Geometry check sheet. Reference: drawing and pictorial views, mm from the part's lowest x, y, z. Round coordinates to 2 decimals unless told otherwise and drop trailing zeros. Order: outer loops, then holes, each group sorted by start corner. A loop starts at its lowest first (then second) coordinate and runs counter-clockwise, first axis right, second up.
(1) Cross-section at A-A on y = 10.5. Enter the section's corners in (x, z), and give its area (3 significant figures).
(2) Cross-section at B-B on x = 11.5. Enter the section's corners in (y, z), and give its area (3 significant figures).
(3) Thickness scan on L1, parallel to X at y = 22, z = 55; L2, parallel to Y at x = 54, z = 206.5. Record the ranges inside material, lowest first.
(4) Draft check along Y on the marked faces 1, 2, 3 and 4. Enter one of: pulls with the +Y half, pulls with the -Y half, needs draft (parallel to the pull), parting line crosses it, or undercut.
(5) Cross-section at C-C on z = 185.5. Enter the section's corners in (x, y), and give its area (3 significant figures).
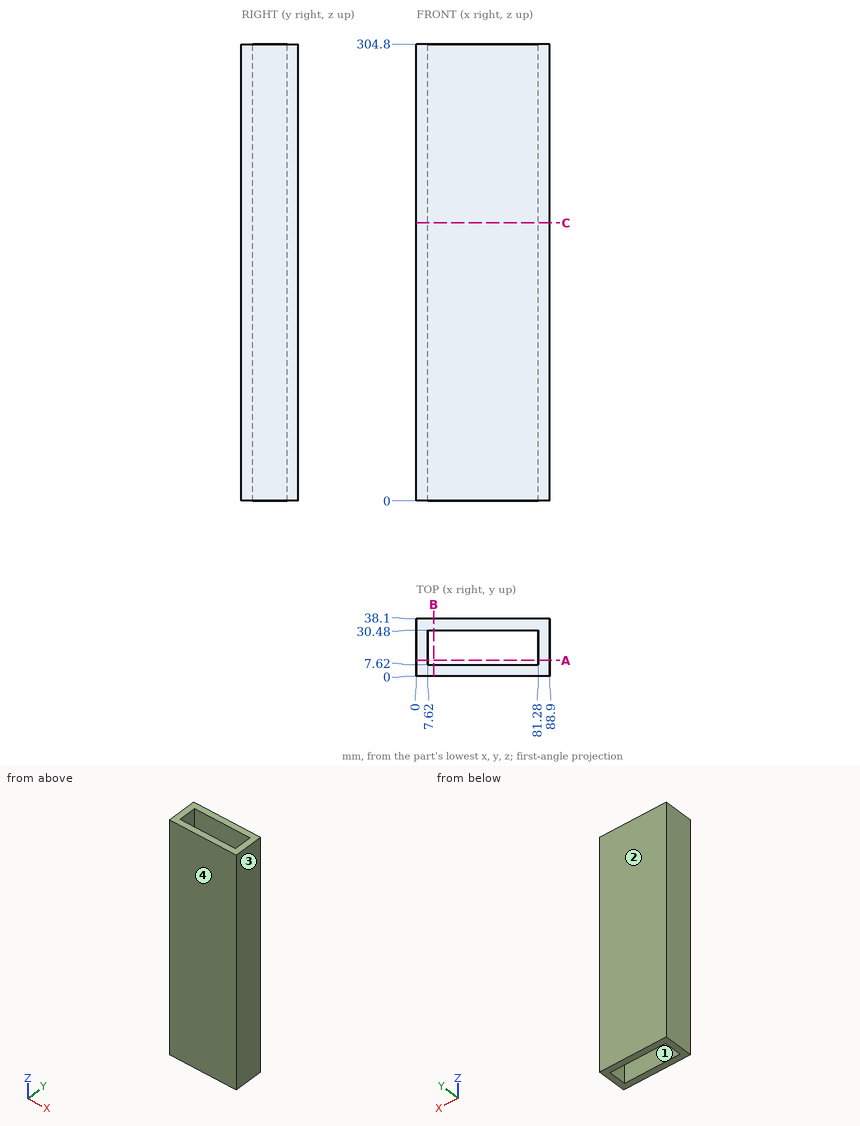
Found:
1. outline: (0, 0) - (7.62, 0) - (7.62, 304.8) - (0, 304.8) - close; (81.28, 0) - (88.9, 0) - (88.9, 304.8) - (81.28, 304.8) - close
1. area: 4,650 mm2
2. outline: (0, 0) - (7.62, 0) - (7.62, 304.8) - (0, 304.8) - close; (30.48, 0) - (38.1, 0) - (38.1, 304.8) - (30.48, 304.8) - close
2. area: 4,650 mm2
3. L1: x = 0 to 7.62, 81.28 to 88.9
3. L2: y = 0 to 7.62, 30.48 to 38.1
4. face 1: undercut
4. face 2: pulls with the +Y half
4. face 3: needs draft
4. face 4: pulls with the -Y half
5. outline: (0, 0) - (88.9, 0) - (88.9, 38.1) - (0, 38.1) - close; hole (7.62, 7.62) - (81.28, 7.62) - (81.28, 30.48) - (7.62, 30.48) - close
5. area: 1,700 mm2
